Design review of the part built by this model. Coordinates are the model's own, in mm. A direction names the side the tool comes from. Round coordinates to 2 decimals unless told otherwise and drop trailing zeros. Loops run counter-clockwise (first coordinate to the right, second up) from the corner with the lowest first, then second, coordinate; pieces in that order, holes last. Notation, with made-up numbers: (15, 19) - (53, 19) arc R14 ccw to (53, 29) - close; hole circle Ø3 at (-12, -29). An arc over 180 degrees is marked (long way). Use one line per item in the form item = value. Start each with the question number.
(1) Machinability: for faces 5 (the cylindrical face through (88.435, 5.07, 36.75)), 6 (the flat face through (60, 5, 10)), which of the approach directions +Z, -Z, +X, -X, +Y, -Y give a long, thin tool a straight path to every point of the face, cutting with its end or side? Answer none if there is none.
(2) For pin 1 (4.5 mm diameter, centred on x = 34.7, z = -4.5, fed in from +Y); pin 2 (5 mm diameter, centred on x = -68, y = 3.5, fed in from -Z); pin 3 (5 mm diameter, centred on y = 7.5, z = 35.5, fed in from +X); pin 4 (1.5 mm diameter, centred on y = 3.5, z = 65.5, fed in from -X), all flat-tipped, find the tip position at first contact; note any pin that passes through.
(3) We need section A-A, the plane x = 0. Write out the cut boundary in (y, z).
(4) We need section C-C, the plane y = 5.25. Give the number of separate pieces and of enclosed holes in the cut face, then the cut area to 3 significant figures.
(5) We need section D-D, the plane z = 78.5. Write out the cut boundary in (x, y), then the cut area to 3 significant figures.
(6) Wall thickness on probe 1 along X at (y, z) = (2.25, 9.5); probe 2 along Z at (x, y) = (-19.5, 4) (3 decimals); probe 3 along Z at (x, y) = (31.5, 5.25): over which ranges is each line inside the solid? List them lowest first. Write a range as [from, to].
(7) We need section B-B, the plane x = -69. Write out the cut boundary in (y, z).
(8) The part is to be moulded in two halves that separate along X. For faces 1 (the cylindrical face through (36.81, 4.93, -3.16)), 2 (the flat face through (0, 5, 90)), 3 (the flat face through (-63.93, 4.93, 63.35)), 4 (the flat face through (35.04, 4.93, 49.18)), say which applies: released by +X, released by -X, zero draft, split by the parting line, or undercut.
from build123d import *

# Parameters (mm, degrees)
SKETCH1_R           = 2.5
SKETCH1_W           = 42
SKETCH1_H           = 20
BOSS_EXTRUDE1_DEPTH = 10
FILLET1_R           = 20
SKETCH2_R           = 5
CUT_EXTRUDE1_DEPTH  = 128.671453348


with BuildPart() as part:
    # Sketch1 → Boss-Extrude1 (new body)
    with BuildSketch(Plane(origin=(0, 0, 0), x_dir=(1, 0, 0), z_dir=(0, 1, 0))):
        Polygon((-90, -37.279220614), (-37.279220614, -90), (37.279220614, -90), (90, -37.279220614), (90, 37.279220614), (37.279220614, 90), (-37.279220614, 90), (-90, 37.279220614), align=None)
        with Locations(Location((56.922095886, -63.286056916, 0), (0, 0, 270))):
            Circle(SKETCH1_R, mode=Mode.SUBTRACT)
        with Locations(Location((63.286056916, -56.922095886, 0), (0, 0, 270))):
            Circle(SKETCH1_R, mode=Mode.SUBTRACT)
        with Locations(Location((27.718585823, -21.354624792, 0), (0, 0, 270))):
            Circle(SKETCH1_R, mode=Mode.SUBTRACT)
        with Locations(Location((21.354624792, -27.718585823, 0), (0, 0, 270))):
            Circle(SKETCH1_R, mode=Mode.SUBTRACT)
        with Locations(Location((-27.718585823, -21.354624792, 0), (0, 0, 270))):
            Circle(SKETCH1_R, mode=Mode.SUBTRACT)
        with Locations(Location((-21.354624792, -27.718585823, 0), (0, 0, 270))):
            Circle(SKETCH1_R, mode=Mode.SUBTRACT)
        with Locations(Location((-56.922095886, -63.286056916, 0), (0, 0, 270))):
            Circle(SKETCH1_R, mode=Mode.SUBTRACT)
        with Locations(Location((-63.286056916, -56.922095886, 0), (0, 0, 270))):
            Circle(SKETCH1_R, mode=Mode.SUBTRACT)
        with Locations(Location((-34.7, 4.5, 0), (0, 0, 270))):
            Circle(SKETCH1_R, mode=Mode.SUBTRACT)
        with Locations(Location((-34.7, -4.5, 0), (0, 0, 270))):
            Circle(SKETCH1_R, mode=Mode.SUBTRACT)
        with Locations(Location((-85, -4.5, 0), (0, 0, 270))):
            Circle(SKETCH1_R, mode=Mode.SUBTRACT)
        with Locations(Location((-85, 4.5, 0), (0, 0, 270))):
            Circle(SKETCH1_R, mode=Mode.SUBTRACT)
        with Locations(Location((-21.354624792, 27.718585823, 0), (0, 0, 270))):
            Circle(SKETCH1_R, mode=Mode.SUBTRACT)
        with Locations(Location((-27.718585823, 21.354624792, 0), (0, 0, 270))):
            Circle(SKETCH1_R, mode=Mode.SUBTRACT)
        with Locations(Location((-63.286056916, 56.922095886, 0), (0, 0, 270))):
            Circle(SKETCH1_R, mode=Mode.SUBTRACT)
        with Locations(Location((-56.922095886, 63.286056916, 0), (0, 0, 270))):
            Circle(SKETCH1_R, mode=Mode.SUBTRACT)
        with Locations(Location((27.718585823, 21.354624792, 0), (0, 0, 270))):
            Circle(SKETCH1_R, mode=Mode.SUBTRACT)
        with Locations(Location((21.354624792, 27.718585823, 0), (0, 0, 270))):
            Circle(SKETCH1_R, mode=Mode.SUBTRACT)
        with Locations(Location((56.922095886, 63.286056916, 0), (0, 0, 270))):
            Circle(SKETCH1_R, mode=Mode.SUBTRACT)
        with Locations(Location((63.286056916, 56.922095886, 0), (0, 0, 270))):
            Circle(SKETCH1_R, mode=Mode.SUBTRACT)
        with Locations(Location((34.7, -4.5, 0), (0, 0, 270))):
            Circle(SKETCH1_R, mode=Mode.SUBTRACT)
        with Locations(Location((34.7, 4.5, 0), (0, 0, 270))):
            Circle(SKETCH1_R, mode=Mode.SUBTRACT)
        with Locations(Location((85, 4.5, 0), (0, 0, 270))):
            Circle(SKETCH1_R, mode=Mode.SUBTRACT)
        with Locations(Location((85, -4.5, 0), (0, 0, 270))):
            Circle(SKETCH1_R, mode=Mode.SUBTRACT)
        Polygon((34.542166261, -20.400030637), (20.400030637, -34.542166261), (50.098515447, -64.240651071), (64.240651071, -50.098515447), align=None, mode=Mode.SUBTRACT)
        Polygon((-20.400030637, -34.542166261), (-34.542166261, -20.400030637), (-64.240651071, -50.098515447), (-50.098515447, -64.240651071), align=None, mode=Mode.SUBTRACT)
        with Locations((-59.85, 0)):
            Rectangle(SKETCH1_W, SKETCH1_H, mode=Mode.SUBTRACT)
        Polygon((-34.542166261, 20.400030637), (-20.400030637, 34.542166261), (-50.098515447, 64.240651071), (-64.240651071, 50.098515447), align=None, mode=Mode.SUBTRACT)
        Polygon((20.400030637, 34.542166261), (34.542166261, 20.400030637), (64.240651071, 50.098515447), (50.098515447, 64.240651071), align=None, mode=Mode.SUBTRACT)
        with Locations((59.85, 0)):
            Rectangle(SKETCH1_W, SKETCH1_H, mode=Mode.SUBTRACT)
    extrude(amount=BOSS_EXTRUDE1_DEPTH)

    # Fillet1
    fillet1_edges = [part.edges().sort_by_distance(p)[0] for p in [
        (-37.279220614, 5, -90),
        (37.279220614, 5, -90),
        (90, 5, -37.279220614),
        (90, 5, 37.279220614),
        (37.279220614, 5, 90),
        (-37.279220614, 5, 90),
        (-90, 5, 37.279220614),
        (-90, 5, -37.279220614),
    ]]
    fillet(fillet1_edges, radius=FILLET1_R)

    # Sketch2 → Cut-Extrude1 (cut, through all)
    with BuildSketch(Plane(origin=(0, 10, 0), x_dir=(1, 0, 0), z_dir=(0, 1, 0))):
        with Locations(Location((0, 0, 0), (0, 0, 270))):
            Circle(SKETCH2_R)
    extrude(amount=-CUT_EXTRUDE1_DEPTH, mode=Mode.SUBTRACT)


solid = part.part
Data:
q1.face_5 = +Z, +X, +Y, -Y
q1.face_6 = +Y, -Y
q2.pin_1 = through
q2.pin_2 = -61.78
q2.pin_3 = 89.59
q2.pin_4 = -62.53
q3.outline = (0, -90) - (10, -90) - (10, -5) - (0, -5) - close; (0, 5) - (10, 5) - (10, 90) - (0, 90) - close
q4.separate_pieces = 1
q4.enclosed_holes = 31
q4.area = 21,200 mm^2
q5.outline = (-48.78, 0) - (48.78, 0) - (48.78, 10) - (-48.78, 10) - close
q5.area = 976 mm^2
q6.probe_1 = [-90, -80.85], [-38.85, 38.85], [80.85, 90]
q6.probe_2 = [-90, -29.395], [-26.042, 26.042], [29.395, 90]
q6.probe_3 = [-89.84, -45.64], [-23.44, 23.44], [45.64, 89.84]
q7.outline = (0, -58.28) - (10, -58.28) - (10, -10) - (0, -10) - close; (0, 10) - (10, 10) - (10, 58.28) - (0, 58.28) - close
q8.face_1 = undercut
q8.face_2 = zero draft
q8.face_3 = released by -X
q8.face_4 = undercut
